Check sheet for the drawn part. Datum: minimum x, y, z corner. Units: mm. A direction names the side the tool comes from. Coordinates: 2 decimals unless noted, no trailing zeros. Order: outer loops, then holes, each group sorted by start corner. A loop starts at its lowest first (then second) coordinate and runs counter-clockwise, first axis right, second up.
1. Set-up check for the marked faces 1 and 2: record each of +Z, -Z, +X, -X, +Y, -Y from which the full face is reachable in a straight line by a thin tool's end or side.
2. Thickness scan on line 1 (X direction, y = 28.5, z = 139) (3 decimals). Record the ranges inside material, lowest first.
3. Cross-section at B-B (z = 327). Enter the section's corners in (x, y) (3 decimals), then the cut area to 3 significant figures.
4. Cross-section at A-A (y = 12). Enter the section's corners in (x, z) (3 decimals), then the cut area to 3 significant figures.
5. Gauge pin test, flat ends, axial feed: pin 1 Ø3 at (y, z) = (31, 62) entering from -X; pin 2 Ø17.5 at (y, z) = (19, 129) entering from +X (3 decimals); pin 3 Ø2 at (x, z) = (20.5, 188.5) entering from +Y (3 decimals). Record the tip position at first contact, or that the pin passes through.
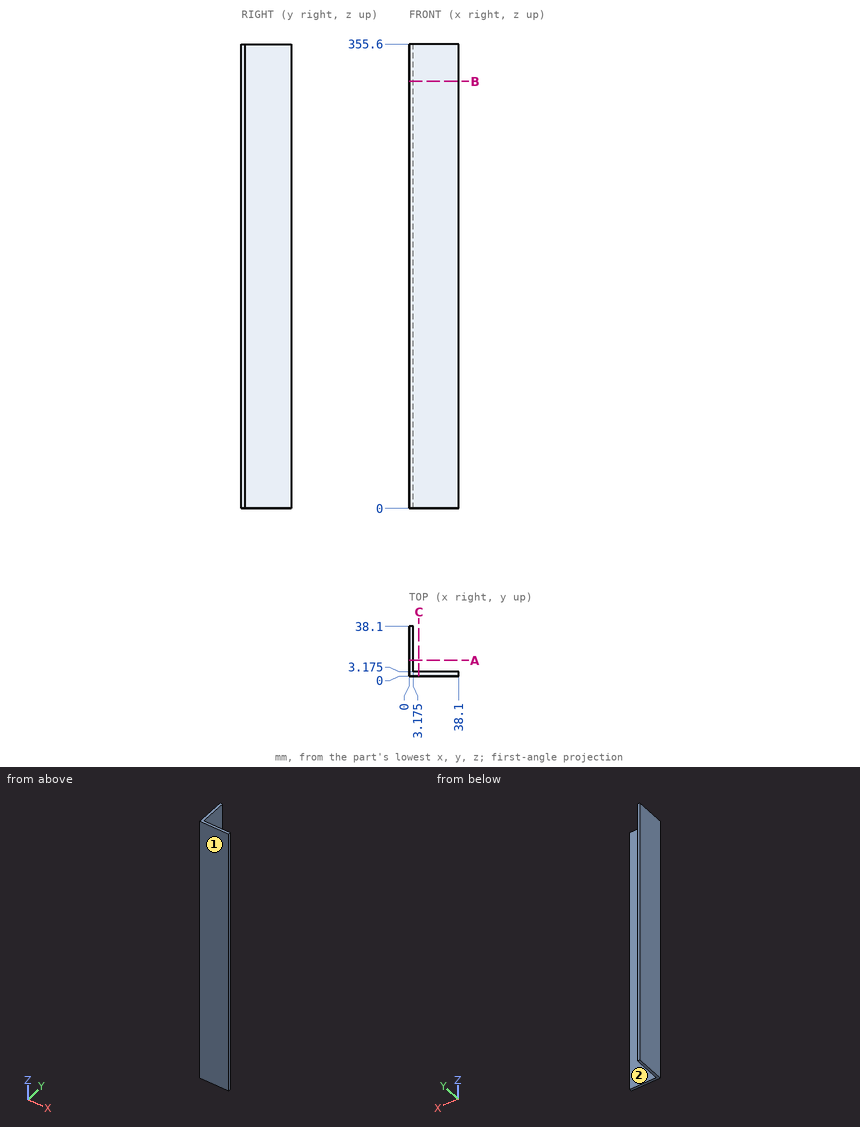
Data:
1. face 1: +Z, -Z, +X, -X, -Y
1. face 2: +Z, -Z, +X, +Y
2. line 1: x = 0 to 3.175
3. outline: (0, 0) - (38.1, 0) - (38.1, 3.175) - (3.175, 3.175) - (3.175, 38.1) - (0, 38.1) - close
3. area: 232 mm2
4. outline: (0, 0) - (3.175, 0) - (3.175, 355.6) - (0, 355.6) - close
4. area: 1,130 mm2
5. pin 1: stops at x = 0
5. pin 2: stops at x = 3.175
5. pin 3: stops at y = 3.175
